Autodesk Inventor part; units mm, degrees
ref_plane "Work Plane1" through (29, 0, 0) normal (0, -1, 0) x (1, 0, 0)
ref_plane "YZ Plane" through (0, 0, 0) normal (1, 0, 0) x (0, 1, 0)
ref_plane "XZ Plane" through (0, 0, 0) normal (0, 1, 0) x (-1, 0, 0)
sketch "Sketch1" plane through (0, 0, 0) normal (0, 0, 1) x (1, 0, 0)
  line L0 (-2.2564, 0) -> (127, 0)
  line L1 (127, 0) -> (127, 4.7625)
  line L2 (127, 4.7625) -> (88.9, 4.7625)
  line L3 (88.9, 4.7625) -> (85.7249, 4.7625)
  line L4 (85.7249, 4.7625) -> (0, 4.7625)
  line L5 (0, 4.7625) -> (0, 7.1501)
  line L6 (0, 7.1501) -> (-9.525, 7.1501)
  line L7 (-9.525, 7.1501) -> (-9.525, 4.5827)
  line L8 (-9.525, 4.5827) -> (-4.9022, 4.5827)
  line L9 (-4.9022, 4.5827) -> (-2.2564, 0)
  line L10 (-36.83, 0) -> (154.305, 0)
  line L11 (0, -1.43) -> (0, 8.5801)
  line L12 (88.9, 4.7625) -> (0, 4.7625) construction
  dimension "d1" = 38.1
  dimension "d2" = 3.1751
  dimension "d3" = 9.525
  dimension "d4" = 4.6228
  dimension "d5" = 60
  dimension "d6" = 9.525
  dimension "d7" = 9.525
  dimension "d8" = 9.1654
  dimension "d9" = 14.3002
  dimension "d26" = 127
revolve "Body" add sketch "Sketch1" angle 360 about axis through (-2.2564, 0, 0) along (1, 0, 0)
sketch "Sketch2" plane through (-9.525, 0, 0) normal (-1, 0, 0) x (0, 0, 1)
  circle A0 centre (0, 0) radius 4.5827
  line L0 (0, -10.0101) -> (0, 10.0101)
  line L1 (-10.0101, 0) -> (10.0101, 0)
  line L2 (4.5827, 0) -> (2.2914, -3.9687)
  line L3 (2.2914, -3.9687) -> (-2.2914, -3.9687)
  line L4 (-2.2914, -3.9687) -> (-4.5827, 0)
  line L5 (-4.5827, 0) -> (-2.2914, 3.9687)
  line L6 (-2.2914, 3.9687) -> (2.2914, 3.9688)
  line L7 (2.2914, 3.9688) -> (4.5827, 0)
extrude "Slot" add sketch "Sketch2" against normal up to next contours L7 A0 | A0 L2 | L6 L0 A0 | A0 L0 L3 | L0 L6 A0 | A0 L3 L0 | L4 A0 | A0 L5
fillet "Fillet1" radius 0.508 1 edges at (-9.525, -7.1501, 0)
thread "Thread"
chamfer "Chamfer1" distance 0.9738 distance2 0.9738 1 edges at (127, -4.7625, 0) measured on face at (127, 0.2765, 1.2306)
ref_plane "Work Plane1" through (29, 0, 0) normal (0, -1, 0) x (1, 0, 0)
fillet "Fillet2" radius 0.1 1 edges at (0, -4.7625, 0)
equation "\"d1\" = GEL"
equation "\"d3\" = KOH"
equation "\"d4\" = INTI"
equation "\"d6\" = GD"
equation "\"d7\" = BDM"
equation "\"d8\" = 1.1547 * SW"
equation "\"d9\" = KOD"
equation "\"d26\" = NLG"
equation "\"d30\" = R"
equation "\"d17\" = RR"
equation "\"d13\" = GEL"
equation "\"d15\" = -0.5 * SPD + 0.5 * GD"
equation "\"d16\" = GUL"
equation "\"GD\" = NND"
equation "\"NLG\" = 127"
equation "\"GEL\" = 38.1"
equation "\"KOD\" = 14.3002"
equation "\"KOH\" = NND"
equation "\"INTI\" = 4.6228"
equation "\"GAL\" = 3.175"
equation "\"GUL\" = 0.97384"
equation "\"BDM\" = NND"
equation "\"SW\" = 7.9375"
equation "\"RR\" = 0.508"
equation "\"SPD\" = GD1"
equation "\"R\" = 0.1"
equation "\"PHH\" = 0.1 * NND"
equation "\"THREADDIA\" = 9.525"
equation "\"FAWI\" = 45deg"
equation "\"NND\" = 9.525"
equation "\"E0\" = 1.155 * SW"
equation "\"FAWI1\" = 30deg"
equation "\"TOA\" = 30deg"
equation "\"GD1\" = 7.57735"
properties part number "Unbrako - 3/8 x 5" material "Steel, Mild"
Can you work these out from the model? Positions are in its coordinate system, mm. A direction names the side the tool comes from. Coordinates: 2 decimals unless noted, no trailing zeros. Loops run counter-clockwise (first coordinate to the right, second up) from the corner with the lowest first, then second, coordinate; pieces in that order, holes last. Notation, with made-up numbers: M 46,40.5 L 82,40.5 A18 cw 82,48.5 Z; hole C 79,21 d9. An arc over 180 degrees is marked long. Put each result on its own line as item: value. Start each with the question number.
(1) Which directions (+Z, -Z, +X, -X, +Y, -Y) give clear straight access to the entire face, cutting with the end or side of a thin tool? Please do faces 1 (the face through (0, 1, -5)), 2 (the face through (-7.07, 1.96, -3.45)), 3 (the face through (-9.525, -4.3, -0.1)).
(2) Imagine slicing it at A-A on x = 107.5. List the corners of the cut face in (y, z) for me (1 decimal).
(3) I need wall thicknesses on probe 1 along X at (y, z) = (1, 6.25) (3 decimals); probe 2 along Y at (x, z) = (65.5, 0.25); probe 3 along Y at (x, z) = (104.5, 1.25). Which ranges of each line are inside material? Lowest first, please.
(4) We'd pull the mould along Y, two halves only. Please class faces 4 (the face through (-4.57, -1.55, 6.98)), 5 (the face through (127, 0, 0)), 6 (the face through (-7.07, -2.01, -3.42)): +Y half, -Y half, draft (parallel to the pull), parting line (faces both ways), or undercut.
(5) Will these pins go through, and if not, where does the flat tip stop? pin 1 Ø6 at (x, y) = (28.5, 1.5) entering from +Z; pin 2 Ø2 at (y, z) = (0, 5.5) entering from +X; pin 3 Ø8 at (x, z) = (103.5, -3.5) entering from -Y.
Worked answers:
1. face 1: +X
1. face 2: -X
1. face 3: +Z, -Z, -X, +Y, -Y
2. outline: C 0,0 d9.5
3. probe 1: x = -9.525 to 0
3. probe 2: y = -4.76 to 4.76
3. probe 3: y = -4.6 to 4.6
4. face 4: parting line
4. face 5: draft
4. face 6: undercut
5. pin 1: stops at z = 4.76
5. pin 2: stops at x = 126.29
5. pin 3: stops at y = -4.76
